Autodesk Inventor part; units mm, degrees
ref_plane "YZ Plane" through (0, 0, 0) normal (1, 0, 0) x (0, 1, 0)
ref_plane "XZ Plane" through (0, 0, 0) normal (0, 1, 0) x (-1, 0, 0)
ref_plane "XY Plane" through (0, 0, 0) normal (0, 0, 1) x (1, 0, 0)
sketch "Esboço1" plane through (0, 0, 0) normal (0, 1, 0) x (-1, 0, 0)
  line L0 (-25.9999, 11.4129) -> (25.9999, -11.4129) construction
  line L1 (28, 11.5) -> (-28, -11.5) construction
  circle A0 centre (0, 0) radius 4
  line L2 (26, 10) -> (-26, 10)
  line L3 (-26, 10) -> (-26, -10)
  line L4 (-26, -10) -> (26, -10)
  line L5 (26, -10) -> (26, 10)
  line L6 (26, 10) -> (-26, -10) construction
  line L7 (-26, 10) -> (26, -10) construction
  line L8 (13, 0) -> (-13, 0)
  circle A1 centre (-13, 0) radius 1
  circle A2 centre (13, 0) radius 1
  line L9 (4.5, 4.5) -> (-4.5, 4.5)
  line L10 (4.5, -4.5) -> (4.5, 4.5)
  line L11 (4.5, 4.5) -> (-4.5, -4.5) construction
  line L12 (-4.5, 4.5) -> (4.5, -4.5) construction
  circle A3 centre (4.5, 4.5) radius 1
  circle A4 centre (4.5, -4.5) radius 1
  circle A5 centre (-4.5, 4.5) radius 1
  circle A6 centre (-4.5, -4.5) radius 1
  line L13 (28, 11.5) -> (-28, 11.5)
  line L14 (-28, 11.5) -> (-28, -11.5)
  line L15 (-28, -11.5) -> (28, -11.5)
  line L16 (28, -11.5) -> (28, 11.5)
  line L17 (28, 11.5) -> (-28, -11.5) construction
  line L18 (-28, 11.5) -> (28, -11.5) construction
  line L19 (26, -10) -> (26, -11.5)
  line L20 (26, 10) -> (26, 11.5)
  line L21 (-26, 10) -> (-26, 11.5)
  line L22 (-26, -10) -> (-26, -11.5)
  dimension "d0" = 54
  dimension "d1" = 23
  dimension "d2" = 8
  dimension "d3" = 52
  dimension "d4" = 20
  dimension "d5" = 26
  dimension "d6" = 2
  dimension "d7" = 2
  dimension "d8" = 9
  dimension "d9" = 9
  dimension "d10" = 2
  dimension "d13" = 9
  dimension "d16" = 9
  dimension "d19" = 56
  dimension "d20" = 23
extrude "Extrusão1" add sketch "Esboço1" along normal blind 34 and the other way blind 2 contours L20 L13 L16 L15 L19 L5 | L3 L22 L15 L14 L13 L21
extrude "Extrusão2" add sketch "Esboço1" along normal blind 5 and the other way blind 2 contours L2 L21 L13 L20 | L19 L15 L22 L4
extrude "Extrusão3" add sketch "Esboço1" against normal blind 2 contours L5 L4 L3 L2
sketch "Esboço3" plane through (-28, -2, -11.5) normal (-1, 0, 0) x (0, 0, 1)
  line L0 (11.5, 2) -> (11.5, 25.4)
  circle A0 centre (11.5, 25.4) radius 4
  line L1 (11.5, 25.4) -> (11.5, 18.4)
  circle A1 centre (11.5, 18.4) radius 1
  circle A2 centre (18.5, 25.4) radius 1
  circle A3 centre (11.5, 32.4) radius 1
  circle A4 centre (4.5, 25.4) radius 1
  line L2 (11.5, 2) -> (-22.5, 2)
  line L3 (7.5, 2) -> (15.5, 2)
  line L4 (11.5, 2) -> (11.5, 36)
  line L5 (-7.4457, 25.4) -> (30.4457, 25.4)
  line L6 (0, 36) -> (0, 7)
  arc A5 (11.5, 36) -> (0, 25.4) centre (12.2417, 23.6571) ccw
  arc A6 (23, 25.4) -> (11.5, 36) centre (10.7583, 23.6571) ccw
  line L7 (0, 0) -> (0, 36)
  line L8 (0, 25.4) -> (0, 36)
  line L9 (0, 36) -> (23, 36)
  line L10 (23, 36) -> (23, 25.4)
  point P0 (-22.5, 2)
  point P1 (11.5, 36)
  point P2 (11.5, 36)
  dimension "d27" = 23.4
  dimension "d28" = 8
  dimension "d29" = 7
  dimension "d30" = 2
  dimension "d33" = 360
  dimension "d39" = 34
  dimension "d40" = 34
extrude "Extrusão4" cut sketch "Esboço3" along normal blind 5.75 and the other way blind 76 contours A1 L0 | L0 A1 | A0 L5 L0 | L0 L5 A0 | L5 A0 L4 | L4 A0 L5 | L5 A4 | A4 L5 | L5 A2 | A2 L5 | L4 A3 | A3 L4
extrude "Extrusão5" cut sketch "Esboço3" along normal blind 5.75 and the other way blind 76 contours L6 L9 A5 | L9 L10 A6
fillet "Arredondamento2" radius 1.5 8 edges at (0, 0, 10) (-26, 0, 0) (0, 0, -10) (26, 0, 0) (0, -2, 11.5) (-28, -2, 0) (0, -2, -11.5) (28, -2, 0)
properties part number "ShotFrame"
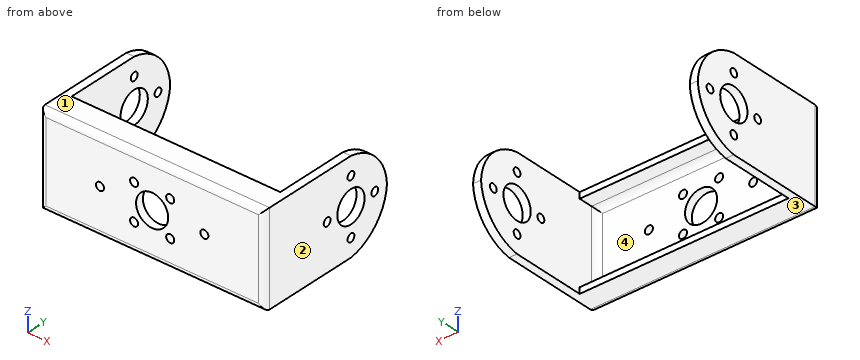
Can you work these out from the model? Positions are in its coordinate system, mm. Face numbers are marked on the shaded views. Coordinates: 2 decimals unless noted, no trailing zeros. Loops run counter-clockwise (first coordinate to the right, second up) from the corner with the lowest first, then second, coordinate; pieces in that order, holes last.
1) Imagine slicing it at B-B on y = 16.4. List the corners of the cut face in (x, z) for me.
2) Imagine slicing it at D-D on z = 7. List the corners of the cut face in (x, y) for me, plus the area to 3 significant figures.
3) Imagine slicing it at A-A on x = 13. List the corners of the cut face in (y, z) for me, plus the area to 3 significant figures.
4) Imagine slicing it at C-C on y = 9.5. List the corners of the cut face in (x, z) for me, plus the area to 3 significant figures.
5) Thinking about a two-plate mould opening in Z: for the marked faces 1, 2, 3 and 4, which applies, pulls with the +Z half, pulls with the -Z half, needs draft (parallel to the pull), parting line crosses it, or undercut?
6) For pin 1 (3 mm diameter, centred on y = 23.4, z = 7, fed in from +X); pin 2 (1.8 mm diameter, centred on x = -4.5, z = -4.5, fed in from -Y); pin 3 (8 mm diameter, centred on x = -21, z = 2, fed in from +Y); pin 4 (3 mm diameter, centred on x = 2.5, z = 4.5, fed in from +Y), each with a flat end and sliding along its axis, tell me the tip position at first contact or that it passes through.
7) I need wall thicknesses on probe 1 along Y at (x, z) = (26.65, 0); probe 2 along X at (y, z) = (15, -3); probe 3 along Z at (x, y) = (22, 3). Which ranges of each line are inside material? Lowest first, please.
Completed:
1. outline: (-28, -11.5) - (-26, -11.5) - (-26, -1) - (-28, -1) - close; (-28, 1) - (-26, 1) - (-26, 11.5) - (-28, 11.5) - close; (26, -11.5) - (28, -11.5) - (28, -1) - (26, -1) - close; (26, 1) - (28, 1) - (28, 11.5) - (26, 11.5) - close
2. outline: (-28, -0.5) arc R1.5 ccw to (-26.5, -2) - (26.5, -2) arc R1.5 ccw to (28, -0.5) - (28, 22.4) - (26, 22.4) - (26, 1.5) arc R1.5 cw to (24.5, 0) - (-24.5, 0) arc R1.5 cw to (-26, 1.5) - (-26, 22.4) - (-28, 22.4) - close; (-28, 24.4) - (-26, 24.4) - (-26, 31.3) - (-28, 31.3) - close; (26, 24.4) - (28, 24.4) - (28, 31.3) - (26, 31.3) - close
2. area: 229 mm2
3. outline: (-2, -10) arc R1.5 ccw to (-0.5, -11.5) - (5, -11.5) - (5, -10) - (1.5, -10) arc R1.5 cw to (0, -8.5) - (0, -1) - (-2, -1) - close; (-2, 1) - (0, 1) - (0, 8.5) arc R1.5 cw to (1.5, 10) - (5, 10) - (5, 11.5) - (-0.5, 11.5) arc R1.5 ccw to (-2, 10) - close
3. area: 57.0 mm2
4. outline: (-28, -11.5) - (-26, -11.5) - (-26, 11.5) - (-28, 11.5) - close; (26, -11.5) - (28, -11.5) - (28, 11.5) - (26, 11.5) - close
4. area: 92.0 mm2
5. face 1: pulls with the +Z half
5. face 2: needs draft
5. face 3: pulls with the -Z half
5. face 4: undercut
6. pin 1: stops at x = 28
6. pin 2: passes through
6. pin 3: stops at y = 0.09
6. pin 4: stops at y = 0
7. probe 1: y = -1.99 to 15.4, 17.4 to 19.4, 27.4 to 29.4, 31.4 to 34
7. probe 2: x = -28 to -26, 26 to 28
7. probe 3: z = -11.5 to -10, 10 to 11.5
